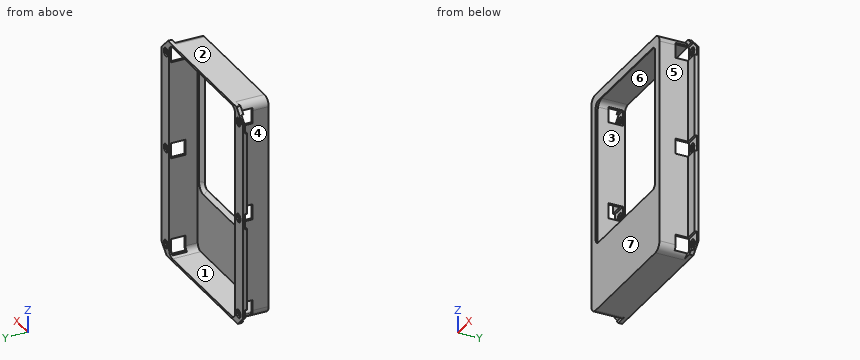
Autodesk Fusion 360 part; units mm, degrees
sketch "Front" plane through (0, 0, 0) normal (0, 1, 0) x (1, 0, 0) in component "2004699A"
  line L0 (-34.4613, 0.7342) -> (100.7673, 0.7342) construction
  line L1 (-34.854, -115.3184) -> (120.0108, -115.3184) construction
  line L2 (39.1093, -14.9122) -> (120.6654, -14.9122) construction
  line L3 (3.575, 24.5274) -> (3.575, -141.9882) construction
  line L4 (78.251, 23.8729) -> (78.251, -119.9956) construction
  line L5 (-16.7886, -108.2138) -> (88.0691, -108.2138) construction
  line L6 (-18.2286, -5.0898) -> (85.3201, -5.0898) construction
  line L7 (-8.6723, -56.6518) -> (96.0546, -56.6518) construction
  line L8 (-24.3813, -113.9722) -> (90.4255, -113.9722) construction
  line L9 (-27.0881, -0.4088) -> (83.5136, -0.4088) construction
  line L10 (10.2552, -130.527) -> (10.2552, 10.1996) construction
  line L11 (71.52, -130.1852) -> (71.52, 12.6775) construction
  line L12 (5.7848, -130.0998) -> (5.7848, 6.3546) construction
  line L13 (83.0008, -137.1267) -> (83.0008, 10.6162) construction
  line L14 (-1.2002, -137.339) -> (-1.2002, 17.644) construction
  line L15 (110.5413, -110.6956) -> (5.7848, -110.6956) construction
  line L16 (110.1974, -34.3178) -> (-2.9547, -34.3178) construction
  line L17 (102.8889, -60.7158) -> (-8.8875, -60.7158) construction
  line L18 (102.459, -52.5878) -> (-11.4669, -52.5878) construction
  line L19 (40.913, -17.1802) -> (40.913, 17.1835) construction
  line L20 (69.6478, 8.6501) -> (89.4046, -11.1067) construction
  line L21 (-5.4342, -8.9542) -> (10.2552, 6.7154) construction
  line L22 (-6.1303, -103.6453) -> (12.6902, -122.4658) construction
  line L23 (73.7302, -117.8806) -> (90.3753, -101.2137) construction
  line L24 (-2.868, -104.1498) -> (87.443, -104.1498) construction
  line L25 (-3.4391, -112.2778) -> (87.0011, -112.2778) construction
  line L26 (-3.1536, -9.1538) -> (86.0732, -9.1538) construction
  line L27 (-3.3677, -1.0258) -> (85.288, -1.0258) construction
  line L28 (10.2552, -110.6956) -> (71.52, -110.6956)
  line L29 (71.52, -110.6956) -> (71.52, -34.3178)
  line L30 (71.52, -34.3178) -> (10.2552, -34.3178)
  line L31 (10.2552, -34.3178) -> (10.2552, -110.6956)
  line L32 (-1.2002, -115.3184) -> (83.0008, -115.3184)
  line L33 (83.0008, -115.3184) -> (83.0008, 0.7342)
  line L34 (83.0008, 0.7342) -> (-1.2002, 0.7342)
  line L35 (-1.2002, 0.7342) -> (-1.2002, -115.3184)
  line L36 (76.0158, -119.9569) -> (76.0158, 9.6762) construction
  line L37 (5.7848, -115.3184) -> (76.0222, -115.3184) construction
  line L38 (76.0222, -115.3184) -> (76.0222, 0.7342) construction
  line L39 (76.0222, 0.7342) -> (5.7848, 0.7342) construction
  line L40 (5.7848, 0.7342) -> (5.7848, -115.3184) construction
  line L41 (76.0222, 0.7342) -> (5.7848, 0.7342)
  line L42 (5.7848, 0.7342) -> (5.7848, -115.3184)
  line L43 (5.7848, -115.3184) -> (76.0222, -115.3184)
  line L44 (76.0222, -115.3184) -> (76.0222, 0.7342)
  line L45 (-1.2002, -108.5588) -> (5.5429, -115.3184)
  line L46 (76.2891, -115.3184) -> (83.0008, -108.585)
  line L47 (77.5637, 0.7342) -> (83.0008, -4.7029)
  line L48 (4.2664, 0.7342) -> (-1.2002, -4.7255)
  point P0 (3.575, -108.2138)
  point P1 (78.251, -108.2138)
  point P2 (78.251, -56.6518)
  point P3 (78.251, -5.0898)
  point P4 (3.575, -5.0898)
  point P5 (3.575, -56.6518)
  dimension "d1" = 1.143
  dimension "d2" = 116.0526
  dimension "d3" = 113.5634
  dimension "d4" = 103.124
  dimension "d5" = 51.562
  dimension "d6" = 74.676
  dimension "d7" = 2.2098
  dimension "d8" = 4.4704
  dimension "d9" = 61.2648
  dimension "d10" = 84.201
  dimension "d11" = 6.985
  dimension "d12" = 76.3778
  dimension "d13" = 4.6228
  dimension "d14" = 100.4062
  dimension "d15" = 37.338
  dimension "d16" = 8.128
  dimension "d17" = 4.064
  dimension "d18" = 3.6322
  dimension "d19" = 3.6322
  dimension "d20" = 3.6322
  dimension "d21" = 3.6322
  dimension "d22" = 4.064
  dimension "d23" = 8.128
  dimension "d25" = 4.064
  dimension "d26" = 8.128
  dimension "d27" = 70.231
extrude "Extrude1" add sketch "Front" against normal blind 17.0434 contours L32 L34 L41 L42 L43 L44 in component "2004699A"
extrude "Extrude2" add sketch "Front" against normal blind 2.0828 contours L32 L34 L35 L42 L45 L48 | L32 L33 L34 L44 L46 L47 in component "2004699A"
fillet "Fillet1" radius 4.318 4 edges at (5.7848, -9.5631, -0.7342) (76.0222, -9.5631, -0.7342) (76.0222, -9.5631, 115.3184) (5.7848, -9.5631, 115.3184) in component "2004699A"
fillet "Fillet2" radius 2.8194 4 edges at (71.52, -8.5217, 110.6956) (10.2552, -8.5217, 110.6956) (71.52, -8.5217, 34.3178) (10.2552, -8.5217, 34.3178) in component "2004699A"
hole "Hole1" at (78.251, 0, 108.2138) at (78.251, 0, 56.6518) at (78.251, 0, 5.0898) at (3.575, 0, 5.0898) at (3.575, 0, 56.6518) at (3.575, 0, 108.2138) direction (0, -1, 0) diameter 4.3434 end through all in component "2004699A"
sketch "Sketch3" plane through (0, 0, 0) normal (0, 1, 0) x (1, 0, 0) in component "2004699A"
  line L0 (88.5571, -114.1754) -> (-29.017, -114.1754) construction
  line L1 (6.9278, -119.135) -> (6.9278, -3.6092) construction
  line L2 (74.8728, -110.975) -> (74.8728, 6.1599) construction
  line L3 (95.5329, -0.4088) -> (-26.782, -0.4088) construction
  line L4 (-34.4613, 0.7342) -> (100.7673, 0.7342) construction
  line L5 (5.7848, -130.0998) -> (5.7848, 6.3546) construction
  line L6 (-34.854, -115.3184) -> (120.0108, -115.3184) construction
  line L7 (76.0158, -119.9569) -> (76.0158, 9.6762) construction
  line L8 (71.6724, -114.1754) -> (10.1282, -114.1754)
  line L9 (6.9278, -110.975) -> (6.9278, -0.4088)
  line L10 (10.1282, -0.4088) -> (71.6724, -0.4088)
  line L11 (74.8728, -3.6092) -> (74.8728, -114.1754)
  arc A0 (74.8728, -3.6092) -> (71.6724, -0.4088) centre (71.6724, -3.6092) ccw
  arc A1 (10.1282, -0.4088) -> (6.9278, -3.6092) centre (10.1282, -3.6092) ccw
  arc A2 (71.6724, -114.1754) -> (74.8728, -110.975) centre (71.6724, -110.975) ccw
  arc A3 (6.9278, -110.975) -> (10.1282, -114.1754) centre (10.1282, -110.975) ccw
  dimension "d37" = 1.143
  dimension "d38" = 1.143
  dimension "d39" = 1.143
  dimension "d40" = 1.143
  dimension "d41" = 3.2004
  dimension "d42" = 3.2004
  dimension "d43" = 3.2004
  dimension "d44" = 3.2004
extrude "Extrude3" cut sketch "Sketch3" against normal blind 14.986 in component "2004699A"
chamfer "Chamfer1" distance 2.032 angle 45 8 edges at (40.8876, -14.986, 34.3178) (11.081, -14.986, 35.1436) (10.2552, -14.986, 72.5067) (11.081, -14.986, 109.8698) (40.8876, -14.986, 110.6956) (70.6942, -14.986, 109.8698) (71.52, -14.986, 72.5067) (70.6942, -14.986, 35.1436) in component "2004699A"
sketch "Sketch4" plane through (83.0008, 0, 0) normal (1, 0, 0) x (0, 1, 0) in component "2004699A"
  line L0 (0, 4.7029) -> (0, 108.585)
  line L1 (0, 108.585) -> (-2.0828, 108.585)
  line L2 (-2.0828, 108.585) -> (-2.0828, 4.7029)
  line L3 (-2.0828, 4.7029) -> (0, 4.7029)
  line L4 (-0.9906, 121.8672) -> (-0.9906, -5.2486) construction
  line L5 (0, 108.2121) -> (-3.3976, 108.2121) construction
  line L6 (0, 56.644) -> (-3.817, 56.644) construction
  line L7 (0, 0) -> (-1.1062, 0) construction
  line L8 (1.8872, 112.2761) -> (-9.9271, 112.2761) construction
  line L9 (1.8112, 104.1481) -> (-10.4595, 104.1481) construction
  line L10 (1.71, 60.708) -> (-9.8241, 60.708) construction
  line L11 (2.1656, 52.58) -> (0.9254, 52.58) construction
  line L12 (0.9254, 52.58) -> (-9.5412, 52.58) construction
  line L13 (0, 5.0822) -> (-6.1548, 5.0822) construction
  line L14 (2.1892, 9.1462) -> (-10.0058, 9.1462) construction
  line L15 (2.6197, 1.0182) -> (-10.581, 1.0182) construction
  line L16 (-8.6106, 122.6091) -> (-8.6106, -10.4565) construction
  line L17 (-8.6106, 60.708) -> (-0.9906, 60.708)
  line L18 (-0.9906, 60.708) -> (-0.9906, 52.58)
  line L19 (-0.9906, 52.58) -> (-8.6106, 52.58)
  line L20 (-8.6106, 52.58) -> (-8.6106, 60.708)
  line L21 (-8.6106, 9.1462) -> (-0.9906, 9.1462)
  line L22 (-0.9906, 9.1462) -> (-0.9906, 1.0182)
  line L23 (-0.9906, 1.0182) -> (-8.6106, 1.0182)
  line L24 (-8.6106, 1.0182) -> (-8.6106, 9.1462)
  line L25 (-8.6106, 112.2761) -> (-0.9906, 112.2761)
  line L26 (-0.9906, 112.2761) -> (-0.9906, 104.1481)
  line L27 (-0.9906, 104.1481) -> (-8.6106, 104.1481)
  line L28 (-8.6106, 104.1481) -> (-8.6106, 112.2761)
  point P0 (0, 119.9956)
  dimension "d48" = 0.9906
  dimension "d49" = 4.064
  dimension "d50" = 8.128
  dimension "d51" = 4.064
  dimension "d52" = 8.128
  dimension "d54" = 4.064
  dimension "d55" = 8.128
  dimension "d56" = 7.62
extrude "Extrude4" cut sketch "Sketch4" against normal through all contours L2 L3 L21 L22 L23 L24 | L2 L3 L21 L22 | L1 L2 L26 L27 | L1 L2 L25 L26 L27 L28 | L2 L17 L19 L20 | L2 L17 L18 L19 in component "2004699A"
component "2004699A" placed x (1, 0, 0) y (0, 1, 0) z (0, 0, 1) at (0, 0, 0)
equation "d41 = 0.171 in - 0.045 in"
equation "d42 = 0.171 in - 0.045 in"
equation "d43 = 0.171 in - 0.045 in"
equation "d44 = 0.171 in - 0.045 in"
Input: part model. Units: mm. Frame: model coordinates. Face numbers are marked on the shaded views. A direction names the side the tool comes from. Coordinates: 2 decimals unless noted, no trailing zeros. Write each loop counter-clockwise with the first axis right and the second up, starting at its lowest first coordinate (ties: lowest second). Pieces come first, ordered by that corner, then holes. Notation, with made-up numbers: (-23.5, 38.5) -> (15.5, 38.5) arc R23 cw to (15.5, 74.5) -> close; hole circle Ø3 at (85, -2). An arc over 180 degrees is marked (long way). Write each question's results on one line, items separated by ' | '.
Item 1: Material intervals for probe 1 along X at (y, z) = (-5.25, 103); probe 2 along Z at (x, y) = (24, -12); probe 3 along Y at (x, z) = (56.5, 19), sorted ascending.
Conclusion:
probe 1: x = 5.78 to 6.93, 74.87 to 76.02 | probe 2: z = -0.73 to 0.41, 114.18 to 115.32 | probe 3: y = -17.04 to -14.99
Item 2: Pin query (flat end, axial travel): pin 1 Ø1.1 at (x, z) = (6.5, 110) entering from +Y; pin 2 Ø1.5 at (y, z) = (-12, 46) entering from -X; pin 3 Ø1.5 at (y, z) = (-3.5, 82.5) entering from +X; pin 4 Ø2.5 at (x, y) = (2, -4) entering from +Z. Return the tip coordinate at first contact, or that it passes through.
Conclusion:
pin 1: stops at y = 0 | pin 2: stops at x = 5.78 | pin 3: stops at x = 76.02 | pin 4: passes through
Item 3: Set-up query: the marked faces 5, 6 and 7. Return all of +Z, -Z, +X, -X, +Y, -Y with unobstructed straight access to the full face (end or side cutting, diameter ignored); none if empty.
Conclusion:
face 5: +Z, -Z, +X, -Y | face 6: +Y | face 7: +Z, -Z, +X, -X, -Y
Item 4: Mould query, pull axis X, two halves, no side actions, for the marked faces 1, 2, 3 and 4. Classes: +X half, -X half, draft (parallel to the pull), parting line (faces both ways), or undercut.
Conclusion:
face 1: undercut | face 2: draft | face 3: undercut | face 4: -X half
Item 5: Section query C-C on y = -12. Return loops of the section in (x, z) (3 decimals), plus the area to 3 significant figures.
Conclusion:
outline: (5.785, 3.584) arc R4.318 ccw to (10.103, -0.734) -> (71.704, -0.734) arc R4.318 ccw to (76.022, 3.584) -> (76.022, 111) arc R4.318 ccw to (71.704, 115.318) -> (10.103, 115.318) arc R4.318 ccw to (5.785, 111) -> close; hole (6.928, 3.609) arc R3.2 ccw to (10.128, 0.409) -> (71.672, 0.409) arc R3.2 ccw to (74.873, 3.609) -> (74.873, 110.975) arc R3.2 ccw to (71.672, 114.175) -> (10.128, 114.175) arc R3.2 ccw to (6.928, 110.975) -> close | area: 414 mm^2
Item 6: Section query D-D on z = 24. Return loops of the section in (x, y).
Conclusion:
outline: (-1.2, -2.08) -> (5.78, -2.08) -> (5.78, -17.04) -> (76.02, -17.04) -> (76.02, -2.08) -> (83, -2.08) -> (83, 0) -> (74.87, 0) -> (74.87, -14.99) -> (6.93, -14.99) -> (6.93, 0) -> (-1.2, 0) -> close
